Work out the finished part from the listing and answer in its coordinate system (mm). A direction names the side the tool comes from. Give positions to 0.01 mm unless a question says otherwise; leave off trailing zeros. Loops run counter-clockwise (first coordinate to the right, second up) from the corner with the lowest first, then second, coordinate; pieces in that order, holes last. Notation, with made-up numbers: M 75,29 L 87,29 A31 cw 87,64 Z; hole C 30.25,-31 d1. An arc over 180 degrees is marked long. Answer as a JSON object with one key per item and string values. Group by question number.
```python
from build123d import *

# Parameters (mm, degrees)
F1_DEPTH = 12.75
F2_R     = 5
F3_R     = 0.75
F4_DEPTH = 1.201
F3_R_2   = 2.05
F5_DEPTH = 0.4
F6_R     = 1.4
F7_DEPTH = 9
F8_R     = 0.8


with BuildPart() as f1:
    # F0 (on Front) → F1 (new body)
    with BuildSketch(Plane.XZ):
        Polygon((5, 0), (0, 0), (-5, 0), (-5, 9), (-15, 9), (-15, -1.2), (0, -1.2), (15, -1.2), (15, 9), (5, 9), align=None)
    extrude(amount=F1_DEPTH)

    # F2
    f2_edges = [f1.edges().sort_by_distance(p)[0] for p in [
        (15, -12.75, 3.9),
        (15, 0, 3.9),
        (-15, -12.75, 3.9),
        (-15, 0, 3.9),
    ]]
    fillet(f2_edges, radius=F2_R)

    # F3 (on face) → F4 (cut, through all)
    with BuildSketch(Plane.XY):
        with Locations((0, -6.375)):
            Circle(F3_R)
    extrude(amount=-F4_DEPTH, mode=Mode.SUBTRACT)

    # F3 (on face) → F5 (cut)
    with BuildSketch(Plane.XY):
        with Locations((0, -6.375)):
            Circle(F3_R_2)
        with Locations((0, -6.375)):
            Circle(F3_R, mode=Mode.SUBTRACT)
    extrude(amount=-F5_DEPTH, mode=Mode.SUBTRACT)

    # F6 (on face) → F7 (cut)
    with BuildSketch(Plane.XY.offset(9)):
        with Locations((11, -6.375)):
            Circle(F6_R)
        with Locations((-11, -6.375)):
            Circle(F6_R)
    extrude(amount=-F7_DEPTH, mode=Mode.SUBTRACT)

    # F8
    f8_edges = [f1.edges().sort_by_distance(p)[0] for p in [
        (-15, -6.375, 9),
        (-13.535534, -1.464466, 9),
        (-13.535534, -11.285534, 9),
        (-7.5, 0, 9),
        (-7.5, -12.75, 9),
        (-5, -6.375, 9),
        (-12.4, -6.375, 9),
        (15, -6.375, 9),
        (13.535534, -1.464466, 9),
        (13.535534, -11.285534, 9),
        (7.5, 0, 9),
        (7.5, -12.75, 9),
        (5, -6.375, 9),
        (9.6, -6.375, 9),
    ]]
    fillet(f8_edges, radius=F8_R)


solid = f1.part
```
Item 1: Find the intervals of material crossed by probe 1 along Y at (x, z) = (0, -0.25) (3 decimals); probe 2 along Y at (x, z) = (10, 1.5); probe 3 along X at (y, z) = (-1, 4.25), in increasing order. Write a range as [from, to].
Item 2: A cutting plane is placed at A-A (x = 0). Determine the outline of the cut face in (y, z) (3 decimals), and give its area (3 significant figures).
Item 3: Given pin 1 Ø2.5 at (y, z) = (-9.5, 4.5) entering from -X; pin 2 Ø1.7 at (x, y) = (0, -6.375) entering from -Z; pin 3 Ø1.4 at (x, y) = (-10.5, -6.5) entering from +Z; pin 4 Ø3.5 at (x, y) = (0, -6.375) entering from +Z, each flat-ended and moving along its own axis, determine where each tip first touches the part or whether it passes through.
Item 4: For a pull along Y with two mould halves and no side action, classify faces 4 (the flat face through (0, -12.75, -1)), 5 (the flat face through (-5, -6, 4)), 6 (the flat face through (11, -6, 0)) as pulls with the +Y half, pulls with the -Y half, needs draft (parallel to the pull), parting line crosses it, or undercut.
Item 5: A cutting plane is placed at C-C (x = 3.5). Determine the outline of the cut face in (y, z).
Item 6: A tool of negligible diameter and unlimited length cuts with its end or side. For faces 1 (the cylindrical face through (-13.57, -11.25, 3.43)), 2 (the flat face through (-11, -6, 0)), 3 (the flat face through (5, -6, 4)), from which of +Z, -Z, +X, -X, +Y, -Y can it reach the whole face along a straight path? Write none if from no direction.
Item 7: A cutting plane is placed at B-B (z = 2.25). Determine the outline of the cut face in (x, y) (3 decimals).
The answers:
{
 "1": {"probe 1": "y = [-12.75, -8.425], [-4.325, 0]", "probe 2": "y = [-12.75, -7.35], [-5.4, 0]", "probe 3": "x = [-13, -5], [5, 13]"},
 "2": {"outline": "M -12.75,-1.2 L -7.125,-1.2 L -7.125,-0.4 L -8.425,-0.4 L -8.425,0 L -12.75,0 Z; M -5.625,-1.2 L 0,-1.2 L 0,0 L -4.325,0 L -4.325,-0.4 L -5.625,-0.4 Z", "area": "12.5 mm^2"},
 "3": {"pin 1": "stops at x = -14.97", "pin 2": "stops at z = -1.2", "pin 3": "stops at z = 0", "pin 4": "stops at z = -0.4"},
 "4": {"face 4": "pulls with the -Y half", "face 5": "needs draft", "face 6": "undercut"},
 "5": {"outline": "M -12.75,-1.2 L 0,-1.2 L 0,0 L -12.75,0 Z"},
 "6": {"face 1": "+Z, -Z, -X, -Y", "face 2": "+Z", "face 3": "+Z, +Y, -Y"},
 "7": {"outline": "M -15,-7.75 A5 ccw -10,-12.75 L -5,-12.75 L -5,0 L -10,0 A5 ccw -15,-5 Z; M 5,-12.75 L 10,-12.75 A5 ccw 15,-7.75 L 15,-5 A5 ccw 10,0 L 5,0 Z; hole C -11,-6.375 d2.8; hole C 11,-6.375 d2.8"}
}
